Input: part model. Units: mm. Frame: model coordinates. A direction names the side the tool comes from. Round coordinates to 2 decimals unless told otherwise and drop trailing zeros. Order: outer loops, then holes, each group sorted by start corner. A loop starts at its lowest first (then second) coordinate and runs counter-clockwise, first axis right, second up.
Item 1: Cut plane D-D on z = 35. Output: boundary loops of the cut face in (x, y).
Item 2: Cut plane A-A on y = 10. Output: boundary loops of the cut face in (x, z).
Item 3: Line query: L1, parallel to Y at x = 1.25, z = 14; L2, parallel to X at y = 4.75, z = 53; L3, parallel to Z at x = -132, y = 12.5. Output: solid intervals per line, ascending.
Item 4: Reachability of faces 5 (the flat face through (-54, 5, 37)), 6 (the flat face through (-54, 15, 37)), 7 (the flat face through (-59.319, 9.93, 36.257)), 8 (the flat face through (-54.9, 9.93, 35.49)) from +Z, -Z, +X, -X, +Y, -Y: full face, straight path, thin tool, end or side. Return the list, or none.
Item 5: First-contact query: pin 1 (6 mm diameter, centred on y = 14, z = 37, fed in from -X); pin 2 (3 mm diameter, centred on x = -57.5, y = 15.5, fed in from +Z); pin 3 (4 mm diameter, centred on y = 15.5, z = 45, fed in from -X). Flat tips, straight axial feed; report the tip coordinate or a pass-through.
Item 6: Cut plane B-B on z = 14. Output: boundary loops of the cut face in (x, y).
Item 7: Cut plane C-C on x = -77. Output: boundary loops of the cut face in (y, z).
Item 8: Mould query, pull axis Y, two halves, no side actions, for faces 1 (the cylindrical face through (1.479, 11.352, 12.526)), 2 (the cylindrical face through (1.48, 10.6, 85.45)), 3 (the flat face through (0, 10, 45)), 4 (the flat face through (-72, 20, -1)). Classes: released by +Y, released by -Y, zero draft, split by the parting line, or undercut.
```python
from build123d import *

# Parameters (mm, degrees)
SALIENTE_EXTRUIR1_DEPTH = 20
CROQUIS2_R              = 2
CORTAR_EXTRUIR1_DEPTH   = 20
CORTAR_EXTRUIR2_DEPTH   = 5
CORTAR_EXTRUIR3_DEPTH   = 5


with BuildPart() as part:
    # Croquis1 → Saliente-Extruir1 (new body)
    with BuildSketch(Plane(origin=(0, 0, 0), x_dir=(1, 0, 0), z_dir=(0, 1, 0))):
        Polygon((3, -92), (3, 3), (-147, 3), (-147, 0), (0, 0), (0, -92), align=None)
        Polygon((-111.362752101, 0), (-117, 0), (0, -73.543441101), (0, -70), align=None)
    extrude(amount=SALIENTE_EXTRUIR1_DEPTH)

    # Croquis2 → Cortar-Extruir1 (cut)
    with BuildSketch(Plane.ZY):
        with Locations((83.543441101, 10)):
            Circle(CROQUIS2_R)
        with Locations((14, 10)):
            Circle(CROQUIS2_R)
    extrude(amount=-CORTAR_EXTRUIR1_DEPTH, mode=Mode.SUBTRACT)

    # Croquis3 → Cortar-Extruir2 (cut)
    with BuildSketch(Plane.XZ):
        Polygon((0, 70), (0, 73.543441101), (-117, 0), (-111.362752101, 0), align=None)
    extrude(amount=-CORTAR_EXTRUIR2_DEPTH, mode=Mode.SUBTRACT)

    # Croquis4 → Cortar-Extruir3 (cut)
    with BuildSketch(Plane(origin=(0, 20, 0), x_dir=(1, 0, 0), z_dir=(0, 1, 0))):
        Polygon((0, -73.543441101), (0, -70), (-111.362752101, 0), (-117, 0), align=None)
    extrude(amount=-CORTAR_EXTRUIR3_DEPTH, mode=Mode.SUBTRACT)


solid = part.part
```
From the geometry:
1. outline: (-61.32, 5) - (-55.68, 5) - (-55.68, 15) - (-61.32, 15) - close; (0, 0) - (3, 0) - (3, 20) - (0, 20) - close
2. outline: (-147, -3) - (3, -3) - (3, 12) - (0, 12) - (0, 0) - (-111.36, 0) - (0, 70) - (0, 16) - (3, 16) - (3, 81.54) - (0, 81.54) - (0, 73.54) - (-117, 0) - (-147, 0) - close; (0, 85.54) - (3, 85.54) - (3, 92) - (0, 92) - close
3. L1: y = 0 to 8, 12 to 20
3. L2: x = 0 to 3
3. L3: z = -3 to 0
4. face 5: +Z, -X, -Y
4. face 6: +Z, -X, +Y
4. face 7: +Z, -X, +Y, -Y
4. face 8: +Y, -Y
5. pin 1: stops at x = -62.91
5. pin 2: stops at z = 38.29
5. pin 3: stops at x = -48.49
6. outline: (-94.73, 5) - (-89.09, 5) - (-89.09, 15) - (-94.73, 15) - close; (0, 0) - (3, 0) - (3, 8) - (0, 8) - close; (0, 12) - (3, 12) - (3, 20) - (0, 20) - close
7. outline: (0, -3) - (20, -3) - (20, 0) - (0, 0) - close; (5, 21.6) - (15, 21.6) - (15, 25.14) - (5, 25.14) - close
8. face 1: undercut
8. face 2: undercut
8. face 3: zero draft
8. face 4: released by +Y
